Can you work these out from the model? Positions are in its coordinate system, mm. A direction names the side the tool comes from. Coordinates: 2 decimals unless noted, no trailing zeros. Order: outer loops, then holes, each group sorted by start corner. A loop starts at its lowest first (then second) coordinate and runs counter-clockwise, first axis right, second up. Notation, with made-up numbers: (-14, 66) - (4, 66) arc R23 cw to (4, 80) - close; hole circle Ø2 at (34.5, 85.25). An arc over 180 degrees is marked (long way). Use a Markdown table: item, result. Add a question column.
(1) I want a section at B-B (y = 33.5). List the corners of the cut face in (x, z) for me, and give its area (3 significant figures).
(2) We'd pull the mould along Y, two halves only. Please class faces 3 (the cylindrical face through (45.997, 109.267, 2.465)), 4 (the flat face through (44, 112, 63.5)): pulls with the +Y half, pulls with the -Y half, needs draft (parallel to the pull), parting line crosses it, or undercut.
(3) On a 3-axis mill with a long thin cutter (end or side, diameter ignored), from which of +Z, -Z, +X, -X, +Y, -Y can I reach the whole of each face in a straight line? I mean faces 1 (the cylindrical face through (-5.95, 109.27, 2.46)), 2 (the flat face through (63, 113, 0)). Say none if no direction works.
(4) I want a section at C-C (x = 112). List the corners of the cut face in (y, z) for me.
(5) I want a section at A-A (z = 2). State how many separate pieces and enclosed holes the cut face has, and give its area (3 significant figures).
(6) I want a section at D-D (z = 48.5). List the corners of the cut face in (x, y) for me, and give its area (3 significant figures).
(7) For pin 1 Ø4 at (x, y) = (-4, 115) entering from +Z; pin 2 Ø1.6 at (x, y) = (46.5, 115.5) entering from +Z; pin 3 Ø4.5 at (x, y) = (-14.12, 115.66) entering from +Z; pin 4 Ø2 at (x, z) = (12, 18.5) entering from -Y, each with a flat end and sliding along its axis, tell me the tip position at first contact or that it passes through.
(8) If I drill on L1, parallel to X at y = 97, z = 42.5; L2, parallel to Y at x = 64, z = 40; L3, parallel to Z at x = 57, y = 68, over which ranges is the centre line in solid material (lowest first)? Write a range as [from, to].
```python
from build123d import *

# Parameters (mm, degrees)
SKETCH5_W           = 153.063311942
SKETCH5_H           = 144.779998932
BOSS_EXTRUDE4_DEPTH = 63.5
FILLET1_R           = 38.1
FILLET2_R           = 2.54
SHELL3_T            = 2.54
SKETCH7_R           = 6.35
BOSS_EXTRUDE5_DEPTH = 5
SKETCH8_R           = 2.625
CUT_EXTRUDE1_DEPTH  = 5
BOSS_EXTRUDE6_DEPTH = 6
FILLET3_R           = 6.35
SKETCH10_R          = 2.625
CUT_EXTRUDE2_DEPTH  = 58.5


with BuildPart() as part:
    # Sketch5 → Boss-Extrude4 (new body)
    with BuildSketch(Plane.XY):
        with Locations((56.058995854, 50.442319529)):
            Rectangle(SKETCH5_W, SKETCH5_H)
    extrude(amount=BOSS_EXTRUDE4_DEPTH)

    # Fillet1
    fillet1_edges = [part.edges().sort_by_distance(p)[0] for p in [
        (-20.472660117, -21.947679937, 31.75),
    ]]
    fillet(fillet1_edges, radius=FILLET1_R)

    # Fillet2
    fillet2_edges = [part.edges().sort_by_distance(p)[0] for p in [
        (132.590651825, -21.947679937, 31.75),
    ]]
    fillet(fillet2_edges, radius=FILLET2_R)

    # Shell3
    shell3_openings = [part.faces().sort_by_distance(p)[0] for p in [
        (57.024076911, 51.357711543, 63.5),
    ]]
    offset(amount=SHELL3_T, openings=shell3_openings, kind=Kind.INTERSECTION)

    # Sketch7 → Boss-Extrude5 (add)
    with BuildSketch(Plane.XY):
        with Locations((62.994650422, 112.820200594)):
            Circle(SKETCH7_R)
        with Locations((123.954650422, 111.804200594)):
            Circle(SKETCH7_R)
        with Locations((64.011650422, 22.578200594)):
            Circle(SKETCH7_R)
        with Locations((124.970650422, 22.396200594)):
            Circle(SKETCH7_R)
        with Locations((-4.569349914, 115.466318873)):
            Circle(SKETCH7_R)
        with Locations((47.373650086, 115.466318873)):
            Circle(SKETCH7_R)
        with Locations((-4.694349914, 15.752318873)):
            Circle(SKETCH7_R)
        with Locations((47.373650086, 15.771318873)):
            Circle(SKETCH7_R)
    extrude(amount=BOSS_EXTRUDE5_DEPTH)

    # Sketch8 → Cut-Extrude1 (cut)
    with BuildSketch(Plane.XY.offset(5)):
        with Locations((-4.694349914, 15.752318873)):
            Circle(SKETCH8_R)
        with Locations((47.373650086, 15.771318873)):
            Circle(SKETCH8_R)
        with Locations((64.011650422, 22.578200594)):
            Circle(SKETCH8_R)
        with Locations((124.970650422, 22.396200594)):
            Circle(SKETCH8_R)
        with Locations((47.373650086, 115.466318873)):
            Circle(SKETCH8_R)
        with Locations((-4.569349914, 115.466318873)):
            Circle(SKETCH8_R)
        with Locations((62.994650422, 112.820200594)):
            Circle(SKETCH8_R)
        with Locations((123.954650422, 111.804200594)):
            Circle(SKETCH8_R)
    extrude(amount=-CUT_EXTRUDE1_DEPTH, mode=Mode.SUBTRACT)

    # Sketch9 → Boss-Extrude6 (add)
    with BuildSketch(Plane.XY.offset(63.5)):
        with BuildLine():
            Line((-6.94761595, 115.657274828), (-6.94761595, 122.832318995))
            Line((-6.94761595, 122.832318995), (-20.472660117, 122.832318995))
            Line((-20.472660117, 122.832318995), (-20.472660117, 115.657274828))
            Line((-20.472660117, 115.657274828), (-20.472660117, 112.316801987))
            ThreePointArc((-20.472660117, 112.316801987), (-12.402234539, 108.691544814), (-6.94761595, 115.657274828))
        make_face()
        with BuildLine():
            Line((33.530571418, 115.657274828), (33.530571418, 122.832318995))
            Line((33.530571418, 122.832318995), (46.230571418, 122.832318995))
            Line((46.230571418, 122.832318995), (46.230571418, 115.657274828))
            ThreePointArc((46.230571418, 115.657274828), (39.880571418, 109.307274828), (33.530571418, 115.657274828))
        make_face()
        with BuildLine():
            Line((68.427420291, 115.710615977), (68.427420291, 122.832318995))
            Line((68.427420291, 122.832318995), (81.127420291, 122.832318995))
            Line((81.127420291, 122.832318995), (81.127420291, 115.710615977))
            ThreePointArc((81.127420291, 115.710615977), (74.777420291, 109.360615977), (68.427420291, 115.710615977))
        make_face()
        with BuildLine():
            Line((126.240651825, 22.296756738), (132.590651825, 22.296756738))
            Line((132.590651825, 22.296756738), (132.590651825, 9.596756738))
            Line((132.590651825, 9.596756738), (126.240651825, 9.596756738))
            ThreePointArc((126.240651825, 9.596756738), (119.890651825, 15.946756738), (126.240651825, 22.296756738))
        make_face()
        with BuildLine():
            Line((-8.880464125, -0.896351485), (-14.122660117, -4.742228331))
            ThreePointArc((-14.122660117, -4.742228331), (-11.33604945, -11.201095808), (-5.089054035, -14.434857763))
            Line((-5.089054035, -14.434857763), (-0.935149274, -10.7884483))
            ThreePointArc((-0.935149274, -10.7884483), (-0.173505163, -2.039817183), (-8.880464125, -0.896351485))
        make_face()
        with BuildLine():
            Line((-14.122660117, 56.792319529), (-20.472660117, 56.792319529))
            Line((-20.472660117, 56.792319529), (-20.472660117, 44.092319529))
            Line((-20.472660117, 44.092319529), (-14.122660117, 44.092319529))
            ThreePointArc((-14.122660117, 44.092319529), (-7.772660117, 50.442319529), (-14.122660117, 56.792319529))
        make_face()
        with BuildLine():
            Line((66.946411889, -15.597679937), (66.946411889, -21.947679937))
            Line((66.946411889, -21.947679937), (79.646411889, -21.947679937))
            Line((79.646411889, -21.947679937), (79.646411889, -15.597679937))
            ThreePointArc((79.646411889, -15.597679937), (73.296411889, -9.247679937), (66.946411889, -15.597679937))
        make_face()
    extrude(amount=-BOSS_EXTRUDE6_DEPTH)

    # Fillet3
    fillet3_edges = [part.edges().sort_by_distance(p)[0] for p in [
        (-20.472660117, 122.832318995, 28.75),
        (132.590651825, 122.832318995, 31.75),
        (-23.012660117, 125.372318995, 30.48),
        (135.130651825, 125.372318995, 30.48),
    ]]
    fillet(fillet3_edges, radius=FILLET3_R)

    # Sketch10 → Cut-Extrude2 (cut)
    with BuildSketch(Plane.XY.offset(63.5)):
        with Locations((-14.122660117, 115.657274828)):
            Circle(SKETCH10_R)
        with Locations((39.880571418, 115.657274828)):
            Circle(SKETCH10_R)
        with Locations((74.777420291, 115.710615977)):
            Circle(SKETCH10_R)
        with Locations((-14.122660117, 50.442319529)):
            Circle(SKETCH10_R)
        with Locations((-5.124288877, -6.016277999)):
            Circle(SKETCH10_R)
        with Locations((73.296411889, -15.597679937)):
            Circle(SKETCH10_R)
        with Locations((126.240651825, 15.946756738)):
            Circle(SKETCH10_R)
    extrude(amount=-CUT_EXTRUDE2_DEPTH, mode=Mode.SUBTRACT)


solid = part.part
```
Answers follow:
| question | item | result |
|---|---|---|
| 1 | outline | (-23.01, -2.54) - (135.13, -2.54) - (135.13, 63.5) - (132.59, 63.5) - (132.59, 0) - (-20.47, 0) - (-20.47, 63.5) - (-23.01, 63.5) - close |
| 1 | area | 724 mm² |
| 2 | face 3 | undercut |
| 2 | face 4 | needs draft |
| 3 | face 1 | none |
| 3 | face 2 | +Z |
| 4 | outline | (-24.49, -2.54) - (125.37, -2.54) - (125.37, 63.5) - (122.83, 63.5) - (122.83, 0) - (-21.95, 0) - (-21.95, 63.5) - (-24.49, 63.5) - close |
| 5 | separate pieces | 9 |
| 5 | enclosed holes | 9 |
| 5 | area | 2,330 mm² |
| 6 | outline | (-23.01, 16.15) arc R40.64 ccw to (17.63, -24.49) - (130.05, -24.49) arc R5.08 ccw to (135.13, -19.41) - (135.13, 119.02) arc R6.35 ccw to (128.78, 125.37) - (-16.66, 125.37) arc R6.35 ccw to (-23.01, 119.02) - close; hole (-20.47, 16.15) arc R38.1 ccw to (17.63, -21.95) - (130.05, -21.95) arc R2.54 ccw to (132.59, -19.41) - (132.59, 116.48) arc R6.35 ccw to (126.24, 122.83) - (-14.12, 122.83) arc R6.35 ccw to (-20.47, 116.48) - close |
| 6 | area | 1,490 mm² |
| 7 | pin 1 | stops at z = 5 |
| 7 | pin 2 | stops at z = 63.5 |
| 7 | pin 3 | stops at z = 0 |
| 7 | pin 4 | stops at y = -24.22 |
| 8 | L1 | x = [-23.01, -20.47], [132.59, 135.13] |
| 8 | L2 | y = [-24.49, -21.95], [122.83, 125.37] |
| 8 | L3 | z = [-2.54, 0] |
